Check sheet for the drawn part. Datum: minimum x, y, z corner. Units: mm. A direction names the side the tool comes from. Give positions to 0.01 mm unless a question says otherwise; leave off trailing zeros. Order: outer loops, then holes, each group sorted by start corner. A loop starts at its lowest first (then second) coordinate and runs counter-clockwise, first axis right, second up.
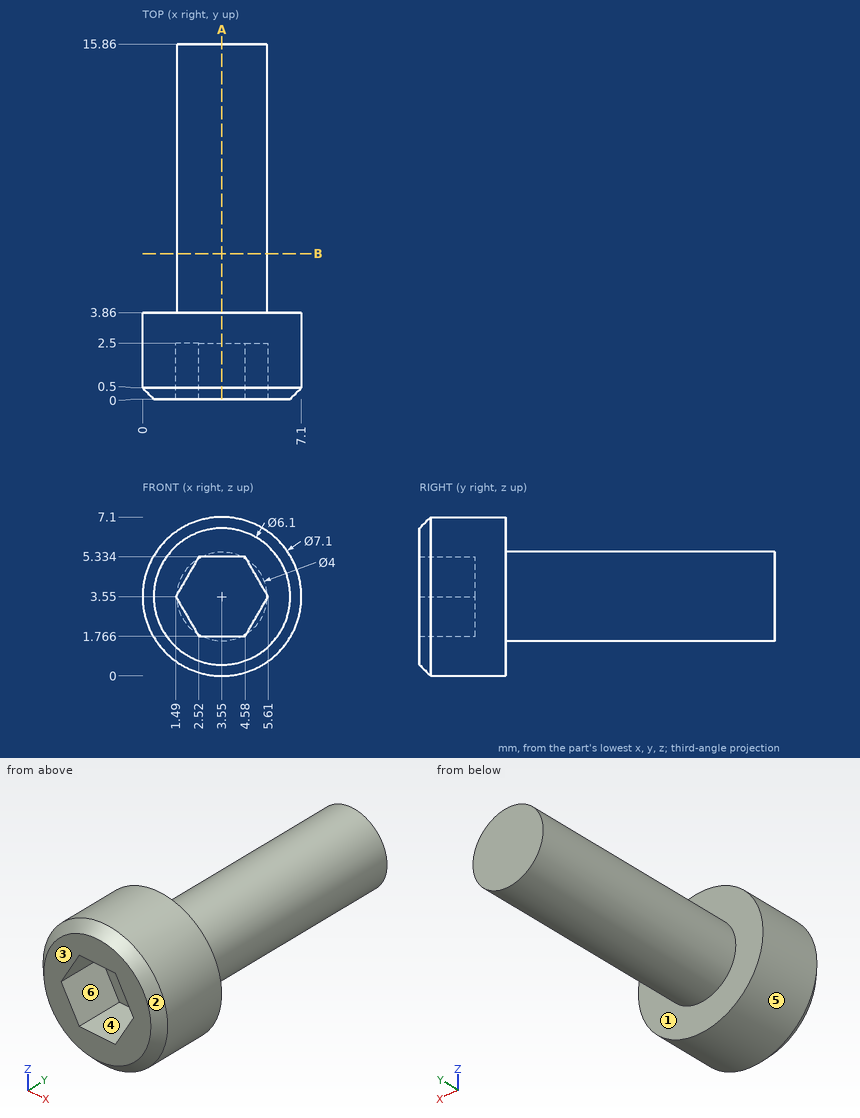
Item 1: Sectioned sample at A-A (x = 3.55). Enter the section's corners in (y, z).
Reported:
outline: (0, 0.5) - (0.5, 0) - (3.86, 0) - (3.86, 1.55) - (15.86, 1.55) - (15.86, 5.55) - (3.86, 5.55) - (3.86, 7.1) - (0.5, 7.1) - (0, 6.6) - (0, 5.33) - (2.5, 5.33) - (2.5, 1.77) - (0, 1.77) - close
Item 2: Scan lines: L1, parallel to Y at x = 1, z = 4; L2, parallel to Z at x = 4.25, y = 2 (1 decimal); L3, parallel to Y at x = 5.25, z = 3. Record each from-to range of solid material in increasing order.
Reported:
L1: y = 0 to 3.86
L2: z = 0.1 to 1.8, 5.3 to 7
L3: y = 2.5 to 15.86
Item 3: Draft check along Z on the marked faces 3, 4, 5 and 6. Enter one of: released by +Z, released by -Z, zero draft, split by the parting line, or undercut.
Reported:
face 3: zero draft
face 4: undercut
face 5: split by the parting line
face 6: undercut
Item 4: Gauge pin test, flat end, axial feed: pin 1 (2 mm diameter, centred on x = 4, y = 9, fed in from -Z). Record the tip position at first contact, or that the pin passes through.
Reported:
pin 1: stops at z = 1.55
Item 5: Set-up check for the marked faces 1 and 2: record each of +Z, -Z, +X, -X, +Y, -Y from which the full face is reachable in a straight line by a thin tool's end or side.
Reported:
face 1: +Y
face 2: -Y
Item 6: Sectioned sample at B-B (y = 6.5). Enter the section's corners in (x, z).
Reported:
outline: circle Ø4 at (3.55, 3.55)
